Design review of the part built by this model. Coordinates are the model's own, in mm. Coordinates: 2 decimals unless noted, no trailing zeros. Write each loop counter-clockwise with the first axis right and the second up, starting at its lowest first coordinate (ties: lowest second). Pieces come first, ordered by that corner, then holes. Notation, with made-up numbers: (56.25, 13.25) -> (60.25, 13.25) arc R10 cw to (60.25, 27.25) -> close; hole circle Ø4 at (-32.5, 6.5). An arc over 180 degrees is marked (long way). Return JSON: item names as keys, results as strings. Group by question number.
from build123d import *

# Parameters (mm, degrees)
F0_W     = 20
F0_H     = 298
F1_DEPTH = 20
F2_T     = -2.5
F3_W     = 5
F3_H     = 5
F4_DEPTH = 1
F5_D     = 4


# Not quite as in the source:
# - a feature names something its author has since deleted; it is built from what else it names


with BuildPart() as f1:
    # F0 (on Right) → F1 (new body)
    with BuildSketch(Plane.YZ):
        Rectangle(F0_W, F0_H)
    extrude(amount=F1_DEPTH)

    # F2
    f2_openings = [f1.faces().sort_by_distance(p)[0] for p in [
        (10, 0, 149),
    ]]
    offset(amount=F2_T, openings=f2_openings)

    # F3 (on face) → F4 (join)
    with BuildSketch(Plane(origin=(0, 0, 0), x_dir=(0, -1, 0), z_dir=(-1, 0, 0))):
        with Locations((12.5, 89)):
            Rectangle(F3_W, F3_H)
        with Locations((-12.5, 89)):
            Rectangle(F3_W, F3_H)
        with Locations((-12.5, -21)):
            Rectangle(F3_W, F3_H)
        with Locations((12.5, -21)):
            Rectangle(F3_W, F3_H)
    extrude(amount=-F4_DEPTH)

    # F5 (through all)
    with Locations(Plane(origin=(0, 0, 0), x_dir=(0, -1, 0), z_dir=(-1, 0, 0))):
        with Locations((-12.5, 89), (12.5, 89), (-12.5, -21), (12.5, -21)):
            Hole(F5_D / 2)


solid = f1.part
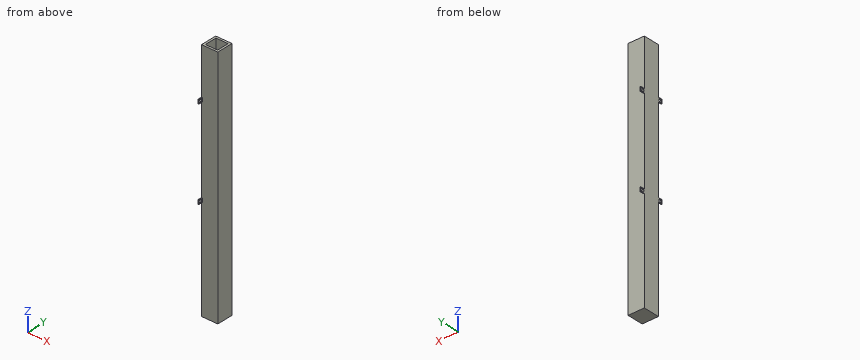
Q1. We need section C-C on y = 2.75. Write out the cut boundary in (x, z), plus the area to 3 significant figures.
Q2. We need section A-A on z = 125.5. Write out the cut boundary in (x, y).
Q3. For P1, Ø4.5, axis at x = 7.5, z = 25, coming from the +Y side; P2, Ø1.5, axis at x = 15, z = -75, coming from the -Y side; P3, Ø3.5, axis at y = 12.5, z = 89, coming from the -X side; P4, Ø1.1, axis at x = 0.5, y = 13.5, coming from the -Z side, all flat-tipped, find the tip position at first contact; note any pin that passes through.
Q4. Wall thickness on L1, parallel to Z at x = 0.5, y = -12.5; L2, parallel to Y at x = 6.75, z = -77; L3, parallel to X at y = 1.25, z = -112.5: over which ranges is each line inside the solid? List them lowest first.
Q5. We need section B-B on x = 8. Write out the cut boundary in (y, z), plus the area to 3 significant figures.
Findings below:
{
 "1": {"outline": "(0, -149) -> (20, -149) -> (20, 149) -> (17.5, 149) -> (17.5, -146.5) -> (2.5, -146.5) -> (2.5, 149) -> (0, 149) -> close", "area": "1,530 mm^2"},
 "2": {"outline": "(0, -10) -> (20, -10) -> (20, 10) -> (0, 10) -> close; hole (2.5, -7.5) -> (17.5, -7.5) -> (17.5, 7.5) -> (2.5, 7.5) -> close"},
 "3": {"P1": "stops at y = 10", "P2": "stops at y = -10", "P3": "passes through", "P4": "stops at z = -23.5"},
 "4": {"L1": "z = -23.5 to -23, -19 to -18.5, 86.5 to 87, 91 to 91.5", "L2": "y = -10 to -7.5, 7.5 to 10", "L3": "x = 0 to 2.5, 17.5 to 20"},
 "5": {"outline": "(-10, -149) -> (10, -149) -> (10, 149) -> (7.5, 149) -> (7.5, -146.5) -> (-7.5, -146.5) -> (-7.5, 149) -> (-10, 149) -> close", "area": "1,530 mm^2"}
}
